```python
from build123d import *

# Parameters (mm, degrees)
F3_DEPTH = 5.08
F4_DEPTH = 25.4


with BuildPart() as f1:
    # F0 (on Front) → F1 (revolve)
    with BuildSketch(Plane.XZ):
        Polygon((9.6376508882, -9.0882862558), (1.2556508882, -9.0882862558), (1.2556508882, -6.6752862558), (0, -6.6752862558), (0, -9.0882862558), (-4.9383663572, -9.0882862558), (-4.9383663572, -10.6122862558), (-16.2532180548, -10.6122862558), (-17.5232180548, -10.6122862558), (-17.5232180548, -11.6282862558), (-16.2532180548, -11.6282862558), (-16.2532180548, -11.0669787973), (0, -11.6282862558), (0, -13.3554862558), (1.778, -13.3554862558), (1.778, -11.6282862558), (10.9076508882, -11.6282862558), (10.9076508882, -10.6122862558), (9.6376508882, -10.6122862558), align=None)
    revolve(axis=Axis((-3.3077835833, 0, -6.6752862558), (-1, 0, 0)))

    # F2 (on face) → F3 (cut)
    with BuildSketch(Plane(origin=(-17.5232180548, 0, 0), x_dir=(0, -1, 0), z_dir=(-1, 0, 0))):
        with BuildLine():
            Line((-3.8987080534, -6.1275230643), (-4.9226176457, -6.1275230643))
            ThreePointArc((-4.9226176457, -6.1275230643), (-4.953, -6.6752862558), (-4.9226176457, -7.2230494473))
            Line((-4.9226176457, -7.2230494473), (-3.8987080534, -7.2230494473))
            ThreePointArc((-3.8987080534, -7.2230494473), (-3.937, -6.6752862558), (-3.8987080534, -6.1275230643))
        make_face()
        with BuildLine():
            ThreePointArc((4.953, -6.6752862558), (4.9453985784, -6.400983685), (4.9226176457, -6.1275230643))
            Line((4.9226176457, -6.1275230643), (3.8987080534, -6.1275230643))
            ThreePointArc((3.8987080534, -6.1275230643), (3.9274153464, -6.4007362662), (3.937, -6.6752862558))
            ThreePointArc((3.937, -6.6752862558), (3.9274153464, -6.9498362454), (3.8987080534, -7.2230494473))
            Line((3.8987080534, -7.2230494473), (4.9226176457, -7.2230494473))
            ThreePointArc((4.9226176457, -7.2230494473), (4.9453985784, -6.9495888266), (4.953, -6.6752862558))
        make_face()
    extrude(amount=-F3_DEPTH, mode=Mode.SUBTRACT)

    # F4 (cut): a face of the model
    f4_faces = [f1.faces().sort_by_distance(p)[0] for p in [
        (1.2556508882, 0, -6.6752862558),
    ]]
    extrude(f4_faces, amount=-F4_DEPTH, mode=Mode.SUBTRACT)


solid = f1.part
```
Source: CAD feature listing. Evaluate the final solid. Frame: model axes, mm. A direction names the side the tool comes from. Give positions to 0.01 mm unless a question says otherwise; leave off trailing zeros. Order: outer loops, then holes, each group sorted by start corner. A loop starts at its lowest first (then second) coordinate and runs counter-clockwise, first axis right, second up. Notation, with made-up numbers: (36, 47) -> (65, 47) arc R31 cw to (65, 85) -> close; hole circle Ø8 at (-8, 51). An arc over 180 degrees is marked (long way). Use a Markdown table: item, result.
Q1. Material intervals for line 1 (Z direction, x = 10.25, y = 0); line 2 (X direction, y = -1.25, z = -11.5); line 3 (Y direction, x = -8.5, z = -4.5), sorted ascending. Write a range as [from, to].
A:
| item | result |
|---|---|
| line 1 | [-11.63, -10.61], [-2.74, -1.72] |
| line 2 | [0, 1.78] |
| line 3 | [-4.12, -3.28], [3.28, 4.12] |
Q2. Section C-C (x = -1.25). Return the cut outline in (y, z).
A:
| item | result |
|---|---|
| outline | circle Ø9.82 at (0, -6.68); hole circle Ø4.83 at (0, -6.68) |
Q3. Section B-B (x = 7.5). Return the cut outline in (y, z), and give its area (3 significant figures).
A:
| item | result |
|---|---|
| outline | circle Ø9.91 at (0, -6.68); hole circle Ø4.83 at (0, -6.68) |
| area | 58.8 mm^2 |
Q4. Pull-direction query (X, two-part tool) for faces 1 (the face through (10.908, 2, -3)), 2 (the face through (0, 0, -12)), 3 (the face through (-16.253, 0.7, -11.2)); classes: +X half, -X half, draft (parallel to the pull), parting line (faces both ways), or undercut.
A:
| item | result |
|---|---|
| face 1 | +X half |
| face 2 | -X half |
| face 3 | undercut |
Q5. Access query for faces 4 (the face through (-15, 4.2, -6.128)), 5 (the face through (-11.319, 3.843, -5.822)), 6 (the face through (-16.879, -0.101, -1.723)), 7 (the face through (-8.013, 2.845, -2.964)), 8 (the face through (6.407, -0.218, -1.727)). Directions: +Z, -Z, +X, -X, +Y, -Y. A direction counts if a zero-diameter tool reaches every point of the face in a straight line with its end or side. Return the directions, or none.
A:
| item | result |
|---|---|
| face 4 | -X, +Y, -Y |
| face 5 | -X |
| face 6 | +Z, -X |
| face 7 | none |
| face 8 | +X |
Q6. Section A-A (y = 0). Return the cut outline in (x, z), and give its area (3 significant figures).
A:
| item | result |
|---|---|
| outline | (-17.52, -11.63) -> (-16.25, -11.63) -> (-16.25, -11.07) -> (0, -11.63) -> (0, -13.36) -> (1.78, -13.36) -> (1.78, -11.63) -> (10.91, -11.63) -> (10.91, -10.61) -> (9.64, -10.61) -> (9.64, -9.09) -> (-4.94, -9.09) -> (-4.94, -10.61) -> (-17.52, -10.61) -> close; (-17.52, -2.74) -> (-4.94, -2.74) -> (-4.94, -4.26) -> (9.64, -4.26) -> (9.64, -2.74) -> (10.91, -2.74) -> (10.91, -1.72) -> (1.78, -1.72) -> (1.78, 0) -> (0, 0) -> (0, -1.72) -> (-16.25, -2.28) -> (-16.25, -1.72) -> (-17.52, -1.72) -> close |
| area | 99.2 mm^2 |
Q7. First-contact query: P1, Ø1.5, axis at x = -5.5, y = -3, coming from the +Z side; P2, Ø4, axis at y = -2, z = -2, coming from the -X side; P3, Ø3, axis at x = 7, y = -1.5, coming from the +Z side; P4, Ø2, axis at x = -7.5, z = -8, coming from the +Y side. Flat tips, straight axial feed; report the tip coordinate or a pass-through.
A:
| item | result |
|---|---|
| P1 | z = -2.48 |
| P2 | x = -17.52 |
| P3 | z = -1.72 |
| P4 | y = 4.69 |
